Part model, mm, in its own coordinate system. A direction names the side the tool comes from. Give positions to 0.01 mm unless a question says otherwise; leave off trailing zeros. Write each loop counter-clockwise with the first axis right and the second up, starting at its lowest first coordinate (ties: lowest second). Pieces come first, ordered by that corner, then holes. Notation, with made-up numbers: (26.25, -13) - (34.25, -13) arc R18 cw to (34.25, 15) - close; hole circle Ø5 at (-10.75, 79.5). An arc over 180 degrees is marked (long way). Answer in a Markdown table with one row per item. Add a question column.
1. Band-saw the part on B-B on y = -38. Write the cut outline in (x, z), plus the area to 4 significant figures.
2. Probe line 1 along Z through (x, y) = (-64.5, 33); line 2 along X through (y, z) = (-46, 35); line 3 along Y through (x, z) = (-1, 17.5). List the from-to ranges inside material, lowest first.
3. Band-saw the part on D-D on y = 9. Write the cut outline in (x, z), plus the area to 3 significant figures.
4. Band-saw the part on A-A on z = 4. Write the cut outline in (x, y), plus the area to 3 significant figures.
5. Which spindle directions (+Z, -Z, +X, -X, +Y, -Y) get a long thin tool onto all of the face, cutting with end or side? Do faces 1 (the cylindrical face through (1.549, -89.987, 24.79)), 2 (the cylindrical face through (-2.14, -321.64, 19.72)). Say none if no direction does.
6. Drop flat-ended pins along their axis: pin 1 Ø8 at (y, z) = (-100, 24.5) entering from +X; pin 2 Ø8 at (y, z) = (-122, 20) entering from +X; pin 3 Ø2 at (y, z) = (-179.5, 5) entering from +X. Give the stop position or say it passes through.
7. Pull direction X, two halves, no side cores. Call faces 3 (the flat face through (-1, 1, 10)), 4 (the cylindrical face through (1.98, 89.98, 4.93)), 5 (the flat face through (-1, -113, 0)): released by +X, released by -X, zero draft, split by the parting line, or undercut.
8. Band-saw the part on C-C on x = -5. Write the cut outline in (y, z).
```python
from build123d import *

# Parameters (mm, degrees)
BOSS_EXTRUDE3_DEPTH = 10
BOSS_EXTRUDE4_DEPTH = 30


with BuildPart() as part:
    # Sketch2 → Boss-Extrude3 (new body)
    with BuildSketch(Plane.XY):
        with BuildLine():
            ThreePointArc((90, 0), (0, 90), (-90, 0))
            Line((-90, 0), (-89.471097217, -9.742831353))
            ThreePointArc((-89.471097217, -9.742831353), (-0.289758357, -89.999533555), (89.406507913, -10.318737459))
            Line((89.406507913, -10.318737459), (90, 0))
        make_face()
        with BuildLine():
            ThreePointArc((89.406507913, -10.318737459), (-0.289758357, -89.999533555), (-89.471097217, -9.742831353))
            Line((-89.471097217, -9.742831353), (-76.448369593, -249.632359432))
            ThreePointArc((-76.448369593, -249.632359432), (-0.525900188, -321.66108657), (75.628074906, -249.877167959))
            Line((75.628074906, -249.877167959), (89.406507913, -10.318737459))
        make_face()
    extrude(amount=BOSS_EXTRUDE3_DEPTH)

    # Sketch3 → Boss-Extrude4 (add)
    with BuildSketch(Plane.XY.offset(10)):
        with BuildLine():
            ThreePointArc((89.406507913, -10.318737459), (-0.289758357, -89.999533555), (-89.471097217, -9.742831353))
            Line((-89.471097217, -9.742831353), (-76.448369593, -249.632359432))
            ThreePointArc((-76.448369593, -249.632359432), (-0.525900188, -321.66108657), (75.628074906, -249.877167959))
            Line((75.628074906, -249.877167959), (89.406507913, -10.318737459))
        make_face()
    extrude(amount=BOSS_EXTRUDE4_DEPTH)


solid = part.part
```
Values:
| question | item | result |
|---|---|---|
| 1 | outline | (-87.94, 0) - (87.81, 0) - (87.81, 40) - (81.58, 40) - (81.58, 10) - (-81.58, 10) - (-81.58, 40) - (-87.94, 40) - close |
| 1 | area | 2,135 mm² |
| 2 | line 1 | z = 0 to 10 |
| 2 | line 2 | x = -87.5 to -77.36, 77.36 to 87.35 |
| 2 | line 3 | y = -321.66 to -89.99 |
| 3 | outline | (-89.55, 0) - (89.55, 0) - (89.55, 10) - (-89.55, 10) - close |
| 3 | area | 1,790 mm² |
| 4 | outline | (-90, 0) - (-76.45, -249.63) arc R76.16 ccw to (75.63, -249.88) - (90, 0) arc R90 ccw to start |
| 4 | area | 62,700 mm² |
| 5 | face 1 | +Z, +Y |
| 5 | face 2 | +Z, -Z, -Y |
| 6 | pin 1 | stops at x = 84.48 |
| 6 | pin 2 | stops at x = 83.21 |
| 6 | pin 3 | stops at x = 79.73 |
| 7 | face 3 | undercut |
| 7 | face 4 | split by the parting line |
| 7 | face 5 | zero draft |
| 8 | outline | (-321.52, 0) - (89.86, 0) - (89.86, 10) - (-89.86, 10) - (-89.86, 40) - (-321.52, 40) - close |
